Could you check a few things on this model? Use its own coordinates, in mm. Round coordinates to 2 decimals unless told otherwise and drop trailing zeros. Write each loop counter-clockwise with the first axis right and the second up, starting at its lowest first coordinate (ties: lowest second). Pieces come first, ordered by that corner, then holes. Notation, with made-up numbers: (45, -10.75) -> (52, -10.75) arc R3 cw to (52, -6.75) -> close; hole circle Ø1 at (-14, -34). An arc over 180 degrees is marked (long way). Answer in a Markdown table with one row per item.
Autodesk Inventor part; units mm, degrees
ref_plane "YZ Plane" through (0, 0, 0) normal (1, 0, 0) x (0, 1, 0)
ref_plane "XZ Plane" through (0, 0, 0) normal (0, 1, 0) x (-1, 0, 0)
ref_plane "XY Plane" through (0, 0, 0) normal (0, 0, 1) x (1, 0, 0)
sketch "Sketch1" plane through (0, 0, 0) normal (0, 0, 1) x (1, 0, 0)
  line L0 (-20, -20) -> (20, -20)
  line L1 (20, -20) -> (20, 20)
  line L2 (20, 20) -> (-20, 20)
  line L3 (-20, 20) -> (-20, -20)
  line L4 (-20, -20) -> (20, 20) construction
  line L5 (20, -20) -> (-20, 20) construction
  point P0 (0, 0)
  dimension "d0" = 40
  dimension "d1" = 40
extrude "Extrusion1" add sketch "Sketch1" along normal blind 5
sketch "Sketch2" plane through (0, 0, 5) normal (0, 0, 1) x (1, 0, 0)
  point P0 (0, 0)
  point P1 (-12, 12)
  point P2 (12, 12)
  point P3 (12, -12)
  point P4 (-12, -12)
  point P5 (0, 0)
  dimension "d4" = 24
  dimension "d5" = 12
  dimension "d6" = 24
  dimension "d7" = 12
hole "Hole1" at (-12, 12, 5) at (12, 12, 5) at (12, -12, 5) at (-12, -12, 5) direction (0, 0, -1) diameter 3 depth 5
hole "Hole2" at (0, 0, 5) direction (0, 0, -1) diameter 6.647 depth 5
fillet "Fillet1" radius 5 4 edges at (20, 20, 2.5) (20, -20, 2.5) (-20, -20, 2.5) (-20, 20, 2.5)
fillet "Fillet2" radius 0.5 8 edges at (18.5355, -18.5355, 5) (20, 0, 5) (18.5355, 18.5355, 5) (0, 20, 5) (-18.5355, 18.5355, 5) (-20, 0, 5) (-18.5355, -18.5355, 5) (0, -20, 5)
properties part number "27" material "Gold"
1) Imagine slicing it at A-A, the plane z = 3.65. Please give me the cut outline in (x, y).
Findings:
| item | result |
|---|---|
| outline | (-20, -15) arc R5 ccw to (-15, -20) -> (15, -20) arc R5 ccw to (20, -15) -> (20, 15) arc R5 ccw to (15, 20) -> (-15, 20) arc R5 ccw to (-20, 15) -> close; hole circle Ø3 at (-12, -12); hole circle Ø3 at (-12, 12); hole circle Ø6.65 at (0, 0); hole circle Ø3 at (12, -12); hole circle Ø3 at (12, 12) |
2) Imagine slicing it at B-B, the plane y = 12. Please give me the cut outline in (x, z).
Findings:
| item | result |
|---|---|
| outline | (-20, 0) -> (-13.5, 0) -> (-13.5, 5) -> (-19.5, 5) arc R0.5 ccw to (-20, 4.5) -> close; (-10.5, 0) -> (10.5, 0) -> (10.5, 5) -> (-10.5, 5) -> close; (13.5, 0) -> (20, 0) -> (20, 4.5) arc R0.5 ccw to (19.5, 5) -> (13.5, 5) -> close |
3) Imagine slicing it at D-D, the plane y = 0. Please give me the cut outline in (x, z), plus the area to 3 significant figures.
Findings:
| item | result |
|---|---|
| outline | (-20, 0) -> (-3.32, 0) -> (-3.32, 5) -> (-19.5, 5) arc R0.5 ccw to (-20, 4.5) -> close; (3.32, 0) -> (20, 0) -> (20, 4.5) arc R0.5 ccw to (19.5, 5) -> (3.32, 5) -> close |
| area | 167 mm^2 |
4) Thinking about a two-plate mould opening in X: for faces 1 (the face through (0, 20, 2)), 2 (the face through (-18, 19, 2)), 3 (the face through (1.27, -3.07, 2.46)), which applies, +X half, -X half, draft (parallel to the pull), parting line (faces both ways), or undercut?
Findings:
| item | result |
|---|---|
| face 1 | draft |
| face 2 | -X half |
| face 3 | undercut |
5) For pin 1 (2.5 mm diameter, centred on x = -12, y = -12, fed in from -Z), with a flat end and sliding along its axis, tell me the tip position at first contact or that it passes through.
Findings:
| item | result |
|---|---|
| pin 1 | passes through |
6) Please list where these lines run through material, in increasing order: line 1 (X direction, y = 12, z = 1.8); line 2 (Y direction, x = 13, z = 3.75).
Findings:
| item | result |
|---|---|
| line 1 | x = -20 to -13.5, -10.5 to 10.5, 13.5 to 20 |
| line 2 | y = -20 to -13.12, -10.88 to 10.88, 13.12 to 20 |
